from build123d import *

# Parameters (mm, degrees)
BOSS_EXTRUDE1_DEPTH = 9
SKETCH2_R           = 2.1
CUT_EXTRUDE1_DEPTH  = 9
CHAMFER1_SIZE       = 2
CHAMFER2_SIZE       = 1.5


with BuildPart() as part:
    # Sketch1 → Boss-Extrude1 (new, symmetric)
    with BuildSketch(Plane.XY):
        Polygon((44, -27.85), (44, 43.65), (-44, 43.65), (-44, -27.85), (-67.5, -27.85), (-67.5, -22.85), (-49, -22.85), (-49, 48.65), (49, 48.65), (49, -22.85), (67.5, -22.85), (67.5, -27.85), align=None)
    extrude(amount=BOSS_EXTRUDE1_DEPTH, both=True)

    # Sketch2 → Cut-Extrude1 (cut, symmetric)
    with BuildSketch(Plane.XZ.offset(27.85)):
        with Locations(Location((55, 0, 0), (0, 0, 270))):
            Circle(SKETCH2_R)
        with Locations(Location((-55, 0, 0), (0, 0, 180))):
            Circle(SKETCH2_R)
    extrude(amount=CUT_EXTRUDE1_DEPTH, both=True, mode=Mode.SUBTRACT)

    # Chamfer1
    chamfer1_edges = [part.edges().sort_by_distance(p)[0] for p in [
        (55, -22.85, 2.1),
        (-52.9, -22.85, 0),
    ]]
    chamfer(chamfer1_edges, length=CHAMFER1_SIZE)

    # Chamfer2
    chamfer2_edges = [part.edges().sort_by_distance(p)[0] for p in [
        (58.25, -22.85, 9),
        (-58.25, -22.85, -9),
        (-49, 12.9, -9),
        (0, 48.65, -9),
        (49, 12.9, -9),
        (58.25, -22.85, -9),
        (49, 12.9, 9),
        (0, 48.65, 9),
        (-67.5, -22.85, 0),
        (-49, -22.85, 0),
        (-49, 48.65, 0),
        (49, 48.65, 0),
        (49, -22.85, 0),
        (67.5, -22.85, 0),
        (-49, 12.9, 9),
        (-58.25, -22.85, 9),
    ]]
    chamfer(chamfer2_edges, length=CHAMFER2_SIZE)


solid = part.part
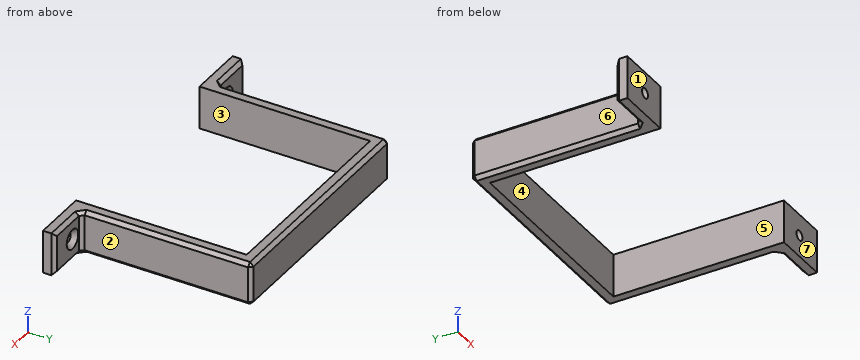
CAD build for the part. Positions are in the model's coordinates, mm. Face numbers are marked on the shaded views. A direction names the side the tool comes from. Give positions to 0.01 mm unless a question says otherwise; leave off trailing zeros. Write each loop counter-clockwise with the first axis right and the second up, starting at its lowest first coordinate (ties: lowest second). Pieces come first, ordered by that corner, then holes. Notation, with made-up numbers: M 31.25,-7.75 L 44.25,-7.75 A31 ccw 44.25,22.25 Z; hole C 55,25.25 d11. An arc over 180 degrees is marked long. Put each result on its own line as item: value. Start each with the question number.
(1) Probe L1, parallel to Z at x = -55, y = -26.45; L2, parallel to X at y = 38.5, z = 3; L3, parallel to Y at x = 1.5, z = 6.25. List the from-to ranges inside material, lowest first.
(2) Band-saw the part on C-C, the plane x = 55. Write the cut outline in (y, z).
(3) Mould opens along X. For the marked faces 4, 5, 6 and 7 say: +X half, -X half, draft (parallel to the pull), parting line (faces both ways), or undercut.
(4) Band-saw the part on B-B, the plane z = 0. Give the number of separate pieces and of enclosed holes in the cut face, and give its area (3 significant figures).
(5) Flat gauge pins, fed straight in: pin 1 Ø6.5 at (x, z) = (55, 0) entering from -Y; pin 2 Ø4.5 at (y, z) = (27, 1) entering from +X; pin 3 Ø1.5 at (x, y) = (50, 3) entering from -Z; pin 4 Ø3 at (y, z) = (-9.5, -1.5) entering from -X. Where does each tip first touch, or does it go through?
(6) Band-saw the part on A-A, the plane y = 37. Write the cut outline in (x, z).
(7) Which spindle directions (+Z, -Z, +X, -X, +Y, -Y) get a long thin tool onto all of the face, cutting with end or side? Do the marked faces 1, 2 and 3. Say none if no direction does.
(8) Band-saw the part on D-D, the plane x = -33.5. Write the cut outline in (y, z).
Response values:
1. L1: z = -9 to -2.1, 2.1 to 9
1. L2: x = -49 to -44, 44 to 49
1. L3: y = 43.65 to 48.65
2. outline: M -27.85,-9 L -24.35,-9 L -22.85,-7.5 L -22.85,-4.1 L -24.85,-2.1 L -27.85,-2.1 Z; M -27.85,2.1 L -24.85,2.1 L -22.85,4.1 L -22.85,7.5 L -24.35,9 L -27.85,9 Z
3. face 4: undercut
3. face 5: undercut
3. face 6: -X half
3. face 7: draft
4. separate pieces: 3
4. enclosed holes: 0
4. area: 1,340 mm2
5. pin 1: stops at y = -27.85
5. pin 2: stops at x = 49
5. pin 3: passes through
5. pin 4: stops at x = -49
6. outline: M -49,-7.5 L -47.5,-9 L -44,-9 L -44,9 L -47.5,9 L -49,7.5 Z; M 44,-9 L 47.5,-9 L 49,-7.5 L 49,7.5 L 47.5,9 L 44,9 Z
7. face 1: +Z, -Z, +X, -X, -Y
7. face 2: +Z, -Z, +X, +Y
7. face 3: +Z, -Z, -Y
8. outline: M 43.65,-9 L 47.15,-9 L 48.65,-7.5 L 48.65,7.5 L 47.15,9 L 43.65,9 Z
